The model under review builds one solid part; all positions refer to its coordinate system, in mm. A direction names the side the tool comes from. Give positions to 0.01 mm unless a question says otherwise; leave off trailing zeros. Loops run counter-clockwise (first coordinate to the right, second up) from the corner with the lowest first, then second, coordinate; pieces in that order, holes last. Notation, with made-up numbers: (-22, 53) -> (17, 53) arc R9 ccw to (17, 65) -> close; hole circle Ø10 at (14.25, 54.25). An arc over 180 degrees is marked (long way). Write each question's results on one line, items separated by ' | '. Start each with the question number.
Q1. We need section B-B (x = 9.5). Write out the cut boundary in (y, z), plus the area to 3 significant figures.
Q2. Machinability: for faces 4 (the face through (11.5, -19, 12)), 5 (the face through (13.5, -6, 12)), 6 (the face through (5, -30.1, 1.5)), 7 (the face through (17.7, -8.36, 1.01)), which of the approach directions +Z, -Z, +X, -X, +Y, -Y give a long, thin tool a straight path to every point of the face, cutting with its end or side? Answer none if there is none.
Q3. Wall thickness on L1, parallel to Y at x = 9.5, z = 1.3; L2, parallel to Y at x = 12.75, z = 3.25; L3, parallel to Z at x = 24, y = -24: over which ranges is each line inside the solid? List them lowest first. Write a range as [from, to].
Q4. Insertion check: pin 1 Ø8 at (y, z) = (-12.5, 3) entering from -X; pin 2 Ø0.5 at (y, z) = (-32.5, 1.5) entering from +X; pin 3 Ø3.5 at (y, z) = (-8.5, 14.5) entering from -X; pin 4 Ø3.5 at (x, z) = (22, 8) entering from +Y. Each pin has a flat end and moves straight along its axis. Give the tip position at first contact, or say it passes through.
Q5. Mouldability with a two-part tool opening along Z and no side actions: class faces 1 (the face through (0, -13, 8)), 2 (the face through (5.67, -6.95, 2)), 3 (the face through (12, -30, 1)) as released by +Z, released by -Z, zero draft, split by the parting line, or undercut.
Q6. We need section A-A (y = -27.5). Write out the cut boundary in (x, z).
Q7. We need section C-C (z = 3.75). Write out the cut boundary in (x, y).
Q8. We need section D-D (x = 21.75). Write out the cut boundary in (y, z).
from build123d import *

# Parameters (mm, degrees)
SZKIC2_W                    = 25
SZKIC2_H                    = 25
DODANIE_WYCI_GNI_CIE1_DEPTH = 2
DODANIE_WYCI_GNI_CIE2_DEPTH = 20
ZAOKR_GLENIE1_R             = 8
WYTNIJ_WYCI_GNI_CIE1_DEPTH  = 20
ZAOKR_GLENIE2_R             = 0.5
WYTNIJ_WYCI_GNI_CIE2_DEPTH  = 20
WYTNIJ_WYCI_GNI_CIE3_DEPTH  = 20
WYTNIJ_WYCI_GNI_CIE4_DEPTH  = 20
ZAOKR_GLENIE3_R             = 0.5
SZKIC14_W                   = 15
SZKIC14_H                   = 10
DODANIE_WYCI_GNI_CIE3_DEPTH = 1
SZKIC13_R                   = 1
WYTNIJ_WYCI_GNI_CIE5_DEPTH  = 1
SFAZOWANIE1_SIZE            = 0.25


with BuildPart() as part:
    # Szkic2 → Dodanie-wyciągnięcie1 (new body)
    with BuildSketch(Plane.XY):
        with Locations((12.5, -12.5)):
            Rectangle(SZKIC2_W, SZKIC2_H)
    extrude(amount=DODANIE_WYCI_GNI_CIE1_DEPTH)

    # Szkic3 → Dodanie-wyciągnięcie2 (add)
    with BuildSketch(Plane.XY.offset(2)):
        Polygon((11.5, 0), (13.5, 0), (13.5, -11.5), (25, -11.5), (25, -13.5), (13.5, -13.5), (13.5, -25), (11.5, -25), (11.5, -13.5), (0, -13.5), (0, -11.5), (11.5, -11.5), align=None)
    extrude(amount=DODANIE_WYCI_GNI_CIE2_DEPTH)

    # Zaokrąglenie1
    zaokr_glenie1_edges = [part.edges().sort_by_distance(p)[0] for p in [
        (0, 0, 1),
        (25, 0, 1),
    ]]
    fillet(zaokr_glenie1_edges, radius=ZAOKR_GLENIE1_R)

    # Szkic7 → Wytnij-wyciągnięcie1 (cut)
    with BuildSketch(Plane.XY.offset(2)):
        Polygon((10.439339828, -13.5), (11.5, -14.560660172), (5.136038969, -20.924621202), (4.075378798, -19.863961031), align=None)
    extrude(amount=-WYTNIJ_WYCI_GNI_CIE1_DEPTH, mode=Mode.SUBTRACT)

    # Zaokrąglenie2
    zaokr_glenie2_edges = [part.edges().sort_by_distance(p)[0] for p in [
        (4.075378798, -19.863961031, 1),
        (10.439339828, -13.5, 1),
        (11.5, -14.560660172, 1),
        (5.136038969, -20.924621202, 1),
    ]]
    fillet(zaokr_glenie2_edges, radius=ZAOKR_GLENIE2_R)

    # Szkic9 → Wytnij-wyciągnięcie2 (cut)
    with BuildSketch(Plane.XY.offset(2)):
        Polygon((11.5, -10.439339828), (10.439339828, -11.5), (4.075378798, -5.136038969), (5.136038969, -4.075378798), align=None)
    extrude(amount=-WYTNIJ_WYCI_GNI_CIE2_DEPTH, mode=Mode.SUBTRACT)

    # Szkic11 → Wytnij-wyciągnięcie3 (cut)
    with BuildSketch(Plane.XY.offset(2)):
        Polygon((13.5, -10.439339828), (14.560660172, -11.5), (20.924621202, -5.136038969), (19.863961031, -4.075378798), align=None)
    extrude(amount=-WYTNIJ_WYCI_GNI_CIE3_DEPTH, mode=Mode.SUBTRACT)

    # Szkic12 → Wytnij-wyciągnięcie4 (cut)
    with BuildSketch(Plane.XY.offset(2)):
        Polygon((14.560660172, -13.5), (13.5, -14.560660172), (19.863961031, -20.924621202), (20.924621202, -19.863961031), align=None)
    extrude(amount=-WYTNIJ_WYCI_GNI_CIE4_DEPTH, mode=Mode.SUBTRACT)

    # Zaokrąglenie3
    zaokr_glenie3_edges = [part.edges().sort_by_distance(p)[0] for p in [
        (5.136038969, -4.075378798, 1),
        (11.5, -10.439339828, 1),
        (10.439339828, -11.5, 1),
        (4.075378798, -5.136038969, 1),
        (13.5, -10.439339828, 1),
        (19.863961031, -4.075378798, 1),
        (20.924621202, -5.136038969, 1),
        (14.560660172, -11.5, 1),
        (14.560660172, -13.5, 1),
        (20.924621202, -19.863961031, 1),
        (19.863961031, -20.924621202, 1),
        (13.5, -14.560660172, 1),
    ]]
    fillet(zaokr_glenie3_edges, radius=ZAOKR_GLENIE3_R)

    # Szkic14 → Dodanie-wyciągnięcie3 (add)
    with BuildSketch(Plane.XY.offset(2)):
        with Locations((12.5, -30)):
            Rectangle(SZKIC14_W, SZKIC14_H)
    extrude(amount=-DODANIE_WYCI_GNI_CIE3_DEPTH)

    # Szkic13 → Wytnij-wyciągnięcie5 (cut)
    with BuildSketch(Plane.XY.offset(2)):
        with Locations((9.5, -27.5)):
            Circle(SZKIC13_R)
        with Locations((15.5, -27.5)):
            Circle(SZKIC13_R)
    extrude(amount=-WYTNIJ_WYCI_GNI_CIE5_DEPTH, mode=Mode.SUBTRACT)

    # Sfazowanie1
    sfazowanie1_edges = [part.edges().sort_by_distance(p)[0] for p in [
        (8.5, -27.5, 2),
        (14.5, -27.5, 2),
    ]]
    chamfer(sfazowanie1_edges, length=SFAZOWANIE1_SIZE)


solid = part.part
Output:
1) outline: (-35, 1) -> (-28.5, 1) -> (-28.5, 1.75) -> (-28.75, 2) -> (-35, 2) -> close; (-26.5, 1) -> (-25, 1) -> (-25, 0) -> (-16.56, 0) -> (-16.56, 2) -> (-26.25, 2) -> (-26.5, 1.75) -> close; (-14.44, 0) -> (-10.56, 0) -> (-10.56, 2) -> (-11.5, 2) -> (-11.5, 22) -> (-13.5, 22) -> (-13.5, 2) -> (-14.44, 2) -> close; (-8.44, 0) -> (0, 0) -> (0, 2) -> (-8.44, 2) -> close | area: 89.5 mm2
2) face 4: +Z, -X, -Y | face 5: +Z, +X, +Y | face 6: +Z, -Z, -X, -Y | face 7: +Z, -Z
3) L1: [-35, -28.5], [-26.5, -16.56], [-14.44, -10.56], [-8.44, 0] | L2: [-25, 0] | L3: [0, 2]
4) pin 1: x = 0 | pin 2: x = 20 | pin 3: x = 11.5 | pin 4: y = -11.5
5) face 1: zero draft | face 2: released by +Z | face 3: released by -Z
6) outline: (5, 1) -> (8.5, 1) -> (8.5, 1.75) -> (8.25, 2) -> (5, 2) -> close; (10.5, 1) -> (14.5, 1) -> (14.5, 1.75) -> (14.25, 2) -> (10.75, 2) -> (10.5, 1.75) -> close; (16.5, 1) -> (20, 1) -> (20, 2) -> (16.75, 2) -> (16.5, 1.75) -> close
7) outline: (0, -13.5) -> (11.5, -13.5) -> (11.5, -25) -> (13.5, -25) -> (13.5, -13.5) -> (25, -13.5) -> (25, -11.5) -> (13.5, -11.5) -> (13.5, 0) -> (11.5, 0) -> (11.5, -11.5) -> (0, -11.5) -> close
8) outline: (-25, 0) -> (-1.56, 0) -> (-1.56, 2) -> (-11.5, 2) -> (-11.5, 22) -> (-13.5, 22) -> (-13.5, 2) -> (-25, 2) -> close
